Source: three-view drawing plus pictorial views. Frame: mm from the lowest corner of the part. A direction names the side the tool comes from. Round coordinates to 2 decimals unless told otherwise and drop trailing zeros. Loops run counter-clockwise (first coordinate to the right, second up) from the corner with the lowest first, then second, coordinate; pieces in that order, holes last. Notation, with made-up numbers: (-10, 77) -> (16, 77) arc R26 cw to (16, 115) -> close; hole circle Ø9 at (-6.5, 70). An arc over 180 degrees is marked (long way). Answer as a JSON object with one key per item and string values. Group by question number.
Item 1: Pin query (flat end, axial travel): pin 1 (12 mm diameter, centred on x = 59, z = 17.5, fed in from +Y); pin 2 (1.5 mm diameter, centred on x = 57, y = 1.5, fed in from -Z). Return the tip coordinate at first contact, or that it passes through.
Item 2: Set-up query: the marked faces 1 and 2. Return all of +Z, -Z, +X, -X, +Y, -Y with unobstructed straight access to the full face (end or side cutting, diameter ignored); none if empty.
Item 3: Section query B-B on z = 46.5. Return loops of the section in (x, y) (3 decimals).
Item 4: Section query D-D on x = 76.2. Return loops of the section in (y, z), and give its area (3 significant figures).
Item 5: Draft query along X for the marked faces 3 and 4. Return one class per face: released by +X, released by -X, zero draft, split by the parting line, or undercut.
Item 6: Material intervals for line 1 (Y direction, x = 10, z = 69); line 2 (Z direction, x = 39.5, y = 5); line 3 (Z direction, x = 76.2, y = 0.9), sorted ascending. Write a range as [from, to].
Item 7: Section query A-A on x = 44.45. Return loops of the section in (y, z) (1 decimal), and give its area (3 significant figures).
Item 8: Section query C-C on z = 10. Return loops of the section in (x, y).
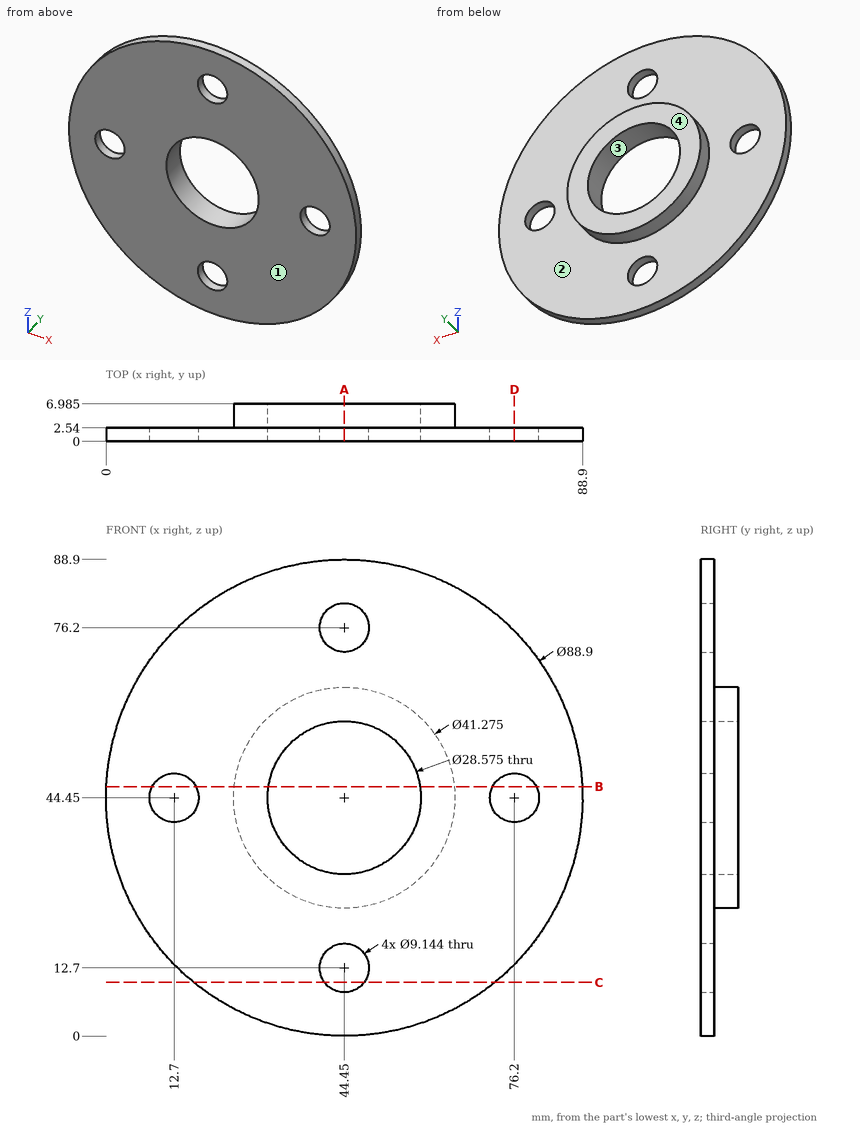
Solved:
{
 "1": {"pin 1": "y = 2.54", "pin 2": "z = 1.59"},
 "2": {"face 1": "+Z, -Z, +X, -X, -Y", "face 2": "+Y"},
 "3": {"outline": "(0.047, 0) -> (8.613, 0) -> (8.613, 2.54) -> (0.047, 2.54) -> close; (16.787, 0) -> (30.31, 0) -> (30.31, 6.985) -> (23.915, 6.985) -> (23.915, 2.54) -> (16.787, 2.54) -> close; (58.59, 0) -> (72.113, 0) -> (72.113, 2.54) -> (64.985, 2.54) -> (64.985, 6.985) -> (58.59, 6.985) -> close; (80.287, 0) -> (88.853, 0) -> (88.853, 2.54) -> (80.287, 2.54) -> close"},
 "4": {"outline": "(0, 13.34) -> (2.54, 13.34) -> (2.54, 39.88) -> (0, 39.88) -> close; (0, 49.02) -> (2.54, 49.02) -> (2.54, 75.56) -> (0, 75.56) -> close", "area": "135 mm²"},
 "5": {"face 3": "undercut", "face 4": "zero draft"},
 "6": {"line 1": "[0, 2.54]", "line 2": "[24.41, 31.05], [57.85, 64.49]", "line 3": "[13.34, 39.88], [49.02, 75.56]"},
 "7": {"outline": "(0, 0) -> (2.5, 0) -> (2.5, 8.1) -> (0, 8.1) -> close; (0, 17.3) -> (2.5, 17.3) -> (2.5, 23.8) -> (7, 23.8) -> (7, 30.2) -> (0, 30.2) -> close; (0, 58.7) -> (7, 58.7) -> (7, 65.1) -> (2.5, 65.1) -> (2.5, 71.6) -> (0, 71.6) -> close; (0, 80.8) -> (2.5, 80.8) -> (2.5, 88.9) -> (0, 88.9) -> close", "area": "163 mm²"},
 "8": {"outline": "(16.36, 0) -> (40.76, 0) -> (40.76, 2.54) -> (16.36, 2.54) -> close; (48.14, 0) -> (72.54, 0) -> (72.54, 2.54) -> (48.14, 2.54) -> close"}
}
